```python
from build123d import *

# Parameters (mm, degrees)
F0_R     = 5.08
F1_DEPTH = 7.62
F2_R     = 1.15124


with BuildPart() as f1:
    # F0 (on Front) → F1 (new body)
    with BuildSketch(Plane.XZ):
        with BuildLine():
            Line((0, 75.388283), (0, 0))
            ThreePointArc((0, 0), (7.123203, -7.123203), (14.246407, 0))
            Line((14.246407, 0), (0, 75.388283))
        make_face()
        with Locations((7.123203, 0)):
            Circle(F0_R, mode=Mode.SUBTRACT)
    extrude(amount=F1_DEPTH)

    # F2
    f2_edges = [f1.edges().sort_by_distance(p)[0] for p in [
        (0, -3.81, 75.388283),
    ]]
    fillet(f2_edges, radius=F2_R)


solid = f1.part
```
Read the model definition and answer for the solid it produces. Units are mm, in the model's axes. Round coordinates to 2 decimals unless told otherwise and drop trailing zeros. Loops run counter-clockwise (first coordinate to the right, second up) from the corner with the lowest first, then second, coordinate; pieces in that order, holes last. Notation, with made-up numbers: (15.5, 71) -> (30.5, 71) arc R18 ccw to (30.5, 81) -> close; hole circle Ø1 at (26, 26). An arc over 180 degrees is marked (long way). One line per item, written item: value.
1) A cutting plane is placed at A-A (x = 5). Determine the outline of the cut face in (y, z).
Answer list:
outline: (-7.62, -6.8) -> (0, -6.8) -> (0, -4.62) -> (-7.62, -4.62) -> close; (-7.62, 4.62) -> (0, 4.62) -> (0, 48.93) -> (-7.62, 48.93) -> close
2) A cutting plane is placed at D-D (x = 1). Determine the outline of the cut face in (y, z), and give its area (3 significant figures).
Answer list:
outline: (-7.62, -3.64) -> (0, -3.64) -> (0, 64.24) -> (-7.62, 64.24) -> close
area: 517 mm²
3) A cutting plane is placed at B-B (y = -2.5). Determine the outline of the cut face in (x, z).
Answer list:
outline: (0, 0) arc R7.12 ccw to (14.25, 0) -> (2.28, 63.31) arc R1.15 ccw to (0, 63.1) -> close; hole circle Ø10.16 at (7.12, 0)
4) Consider L1, parallel to X at y = -6.5, z = 20; L2, parallel to Z at x = 2, y = -3.75; L3, parallel to X at y = -6.25, z = 7.5. Determine where each line is inside the solid, lowest interval first. Write a range as [from, to].
Answer list:
L1: x = [0, 10.47]
L2: z = [-4.95, 63.87]
L3: x = [0, 12.83]
5) A cutting plane is placed at C-C (z = 60). Determine the outline of the cut face in (x, y).
Answer list:
outline: (0, -7.62) -> (2.91, -7.62) -> (2.91, 0) -> (0, 0) -> close
6) The mould has two halves that part along Z. Classify faces 1 (the face through (0, -4, 32)), 2 (the face through (11.969, -3.757, 1.526)), 3 (the face through (1.02, -3.86, 64.24)): pulls with the +Z half, pulls with the -Z half, needs draft (parallel to the pull), parting line crosses it, or undercut.
Answer list:
face 1: needs draft
face 2: undercut
face 3: pulls with the +Z half
